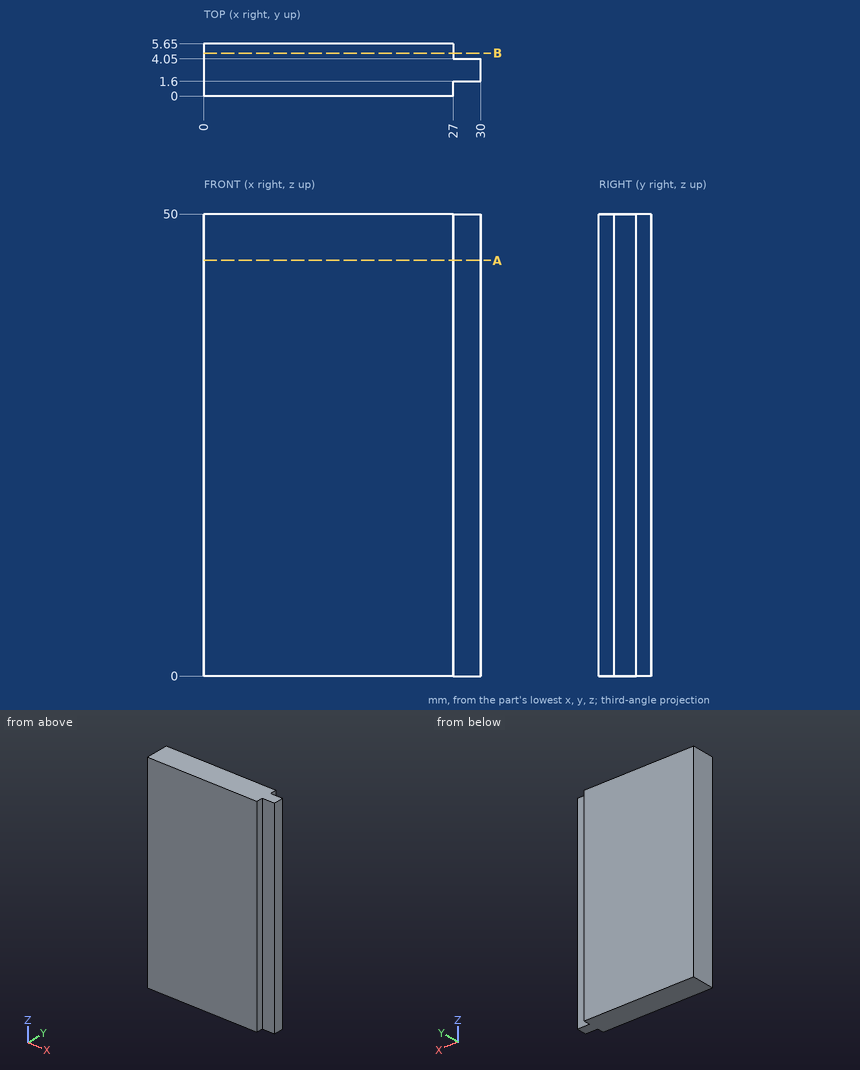
Here's the drawing with two shaded views (mm, measured from the low corner). I have some questions. Give positions to 0.01 mm unless a question says otherwise; leave off trailing zeros. Order: outer loops, then holes, each group sorted by start corner. A loop starts at its lowest first (then second) coordinate and runs counter-clockwise, first axis right, second up. Notation, with made-up numbers: (28.25, -39) -> (37.25, -39) arc R28 ccw to (37.25, -6) -> close; hole circle Ø11 at (-25.5, 15). An arc over 180 degrees is marked (long way). Use a Markdown table: item, result. Add a question column.
Item 1: I need wall thicknesses on line 1 (X direction, y = 0.9, z = 5.5). Which ranges of the line are inside material? Lowest first, please.
Item 2: Imagine slicing it at A-A on z = 45. Please give me the cut outline in (x, y), plus the area to 3 significant figures.
Item 3: Imagine slicing it at B-B on y = 4.65. Please give me the cut outline in (x, z).
Item 4: Will these pins go through, and if not, where does the flat tip stop? pin 1 (1.5 mm diameter, centred on x = 6.5, z = 11, fed in from -Y); pin 2 (2.5 mm diameter, centred on x = 28.5, z = 20, fed in from -Y); pin 3 (0.5 mm diameter, centred on y = 0.5, z = 18.5, fed in from +X).
Data:
| question | item | result |
|---|---|---|
| 1 | line 1 | x = 0 to 27 |
| 2 | outline | (0, 0) -> (27, 0) -> (27, 1.6) -> (30, 1.6) -> (30, 4.05) -> (27, 4.05) -> (27, 5.65) -> (0, 5.65) -> close |
| 2 | area | 160 mm² |
| 3 | outline | (0, 0) -> (27, 0) -> (27, 50) -> (0, 50) -> close |
| 4 | pin 1 | stops at y = 0 |
| 4 | pin 2 | stops at y = 1.6 |
| 4 | pin 3 | stops at x = 27 |
